from build123d import *

# Parameters (mm, degrees)
SKETCH1_R           = 14.2748
SKETCH1_R_2         = 2.032
BOSS_EXTRUDE1_DEPTH = 14.478
CHAMFER1_SIZE       = 0.254


with BuildPart() as part:
    # Sketch1 → Boss-Extrude1 (new body)
    with BuildSketch(Plane.XY):
        Circle(SKETCH1_R)
        with Locations((0, 10.287)):
            Circle(SKETCH1_R_2, mode=Mode.SUBTRACT)
        with Locations((8.908803329, 5.1435)):
            Circle(SKETCH1_R_2, mode=Mode.SUBTRACT)
        with Locations((8.908803329, -5.1435)):
            Circle(SKETCH1_R_2, mode=Mode.SUBTRACT)
        with Locations((0, -10.287)):
            Circle(SKETCH1_R_2, mode=Mode.SUBTRACT)
        with Locations((-8.908803329, -5.1435)):
            Circle(SKETCH1_R_2, mode=Mode.SUBTRACT)
        with Locations((-8.908803329, 5.1435)):
            Circle(SKETCH1_R_2, mode=Mode.SUBTRACT)
        Polygon((-7.332348419, 0), (-3.666174209, -6.35), (3.666174209, -6.35), (7.332348419, 0), (3.666174209, 6.35), (-3.666174209, 6.35), align=None, mode=Mode.SUBTRACT)
    extrude(amount=BOSS_EXTRUDE1_DEPTH)

    # Chamfer1
    chamfer1_edges = [part.edges().sort_by_distance(p)[0] for p in [
        (0, -6.35, 0),
        (5.499261314, -3.175, 0),
        (5.499261314, 3.175, 0),
        (0, 6.35, 0),
        (-5.499261314, 3.175, 14.478),
        (-5.499261314, -3.175, 14.478),
        (0, -6.35, 14.478),
        (5.499261314, -3.175, 14.478),
        (5.499261314, 3.175, 14.478),
        (0, 6.35, 14.478),
        (-14.2748, 0, 0),
        (-2.032, 10.287, 0),
        (-2.032, 10.287, 14.478),
        (6.876803329, 5.1435, 0),
        (6.876803329, 5.1435, 14.478),
        (6.876803329, -5.1435, 0),
        (6.876803329, -5.1435, 14.478),
        (-2.032, -10.287, 0),
        (-2.032, -10.287, 14.478),
        (-10.940803329, -5.1435, 0),
        (-10.940803329, -5.1435, 14.478),
        (-14.2748, 0, 14.478),
        (-10.940803329, 5.1435, 0),
        (-10.940803329, 5.1435, 14.478),
        (-5.499261314, 3.175, 0),
        (-5.499261314, -3.175, 0),
    ]]
    chamfer(chamfer1_edges, length=CHAMFER1_SIZE)


solid = part.part
The listing builds one solid part. Answer for the finished solid, in the listing's coordinates (mm). A direction names the side the tool comes from. Coordinates: 2 decimals unless noted, no trailing zeros. Loops run counter-clockwise (first coordinate to the right, second up) from the corner with the lowest first, then second, coordinate; pieces in that order, holes last. Notation, with made-up numbers: (76.25, 31) -> (89.25, 31) arc R21 cw to (89.25, 37) -> close; hole circle Ø5 at (55, 32). An arc over 180 degrees is marked (long way). Answer in a Markdown table with one row per item. Add a question column.
1. For faces 4 (the flat face through (5.637, 3.193, 0.125)), 5 (the flat face through (6, 3.3, 14.478)), 6 (the flat face through (5.525, 3.131, 7.141)), determine the directions among +Z, -Z, +X, -X, +Y, -Y from which every point of the face is accessible in a straight line to the end or side of a thin tool.
2. The part is cut by section A-A, the plane x = 0. Count the separate pieces of the cut face and the enclosed holes in it, then the cut area to 3 significant figures.
3. The part is cut by section B-B, the plane z = 2.5. Write down the section's boundary in (x, y).
4. Consider line 1 (X direction, y = -6, z = 8); line 2 (X direction, y = 3.5, z = 4.25); line 3 (Y direction, x = 9.5, z = 9). Determine where each line is inside the solid, lowest interval first. Write a range as [from, to].
5. Determine the mould class of faces 1 (the flat face through (6, 3.3, 0)), 2 (the flat face through (-5.58, 3.29, 14.35)), 3 (the cylindrical face through (-14.26, 0.63, 7.14)) for opening direction X: +X half, -X half, draft (parallel to the pull), parting line (faces both ways), or undercut.
6. Flat-ended cylindrical pins translate along their axes: P1, Ø4.5, axis at x = 8.91, y = 5.14, coming from the -Z side; P2, Ø6, axis at x = 8.5, z = 8, coming from the -Y side; P3, Ø3.5, axis at x = -1, z = 8, coming from the +Y side; P4, Ø4, axis at y = 9.5, z = 2.5, coming from the +X side. Find the tip coordinate at first contact, or state that the pin passes through.
Answer below:
| question | item | result |
|---|---|---|
| 1 | face 4 | -Z |
| 1 | face 5 | +Z, +X, -X, +Y, -Y |
| 1 | face 6 | +Z, -Z |
| 2 | separate pieces | 4 |
| 2 | enclosed holes | 0 |
| 2 | area | 111 mm2 |
| 3 | outline | circle Ø28.55 at (0, 0); hole circle Ø4.06 at (-8.91, -5.14); hole circle Ø4.06 at (-8.91, 5.14); hole (-7.33, 0) -> (-3.67, -6.35) -> (3.67, -6.35) -> (7.33, 0) -> (3.67, 6.35) -> (-3.67, 6.35) -> close; hole circle Ø4.06 at (0, -10.29); hole circle Ø4.06 at (0, 10.29); hole circle Ø4.06 at (8.91, -5.14); hole circle Ø4.06 at (8.91, 5.14) |
| 4 | line 1 | [-12.95, -10.75], [-7.07, -3.87], [3.87, 7.07], [10.75, 12.95] |
| 4 | line 2 | [-13.84, -10.1], [-7.71, -5.31], [5.31, 7.71], [10.1, 13.84] |
| 4 | line 3 | [-10.65, -7.09], [-3.2, 3.2], [7.09, 10.65] |
| 5 | face 1 | draft |
| 5 | face 2 | undercut |
| 5 | face 3 | parting line |
| 6 | P1 | z = 0.03 |
| 6 | P2 | y = -13.17 |
| 6 | P3 | y = 14.27 |
| 6 | P4 | x = 12.15 |
